from build123d import *

# Parameters (mm, degrees)
F0_W     = 170
F0_H     = 170
F0_R     = 1.98
F1_DEPTH = 1.57
F2_W     = 155
F2_H     = 27
F3_DEPTH = 39
F4_W     = 155
F4_H     = 30
F5_DEPTH = 38
F6_ANGLE = -90


with BuildPart() as f1:
    # F0 (on Front) → F1 (new body)
    with BuildSketch(Plane.XZ):
        with Locations((85, 85)):
            Rectangle(F0_W, F0_H)
        with Locations((6.35, 4.88)):
            Circle(F0_R, mode=Mode.SUBTRACT)
        with Locations((163.93, 4.88)):
            Circle(F0_R, mode=Mode.SUBTRACT)
        with Locations((6.35, 159.84)):
            Circle(F0_R, mode=Mode.SUBTRACT)
        with Locations((163.93, 147.14)):
            Circle(F0_R, mode=Mode.SUBTRACT)
    extrude(amount=F1_DEPTH)

    # F2 (on face) → F3 (join)
    with BuildSketch(Plane.XZ.offset(1.57)):
        with Locations((92.5, 156.5)):
            Rectangle(F2_W, F2_H)
    extrude(amount=F3_DEPTH)

    # F4 (on face) → F5 (join)
    with BuildSketch(Plane.XZ.offset(1.57)):
        with Locations((92.5, 15)):
            Rectangle(F4_W, F4_H)
    extrude(amount=F5_DEPTH)


with BuildPart() as f1_1:
    # F6: moved
    add(f1.part.rotate(Axis((0, -0.785, 0), (0, 1, 0)), F6_ANGLE))


with BuildPart() as f1_2:
    # F7: moved
    add(f1_1.part.moved(Location((170, 0, 0))))


solid = f1_2.part
Check sheet for the modelled part. Datum: model origin and axes. Units: mm. A direction names the side the tool comes from. Give positions to 0.01 mm unless a question says otherwise; leave off trailing zeros. Write each loop counter-clockwise with the first axis right and the second up, starting at its lowest first coordinate (ties: lowest second). Pieces come first, ordered by that corner, then holes. Notation, with made-up numbers: (19.25, 76) -> (45.25, 76) arc R11 ccw to (45.25, 89) -> close; hole circle Ø1 at (-4.75, 50). An arc over 180 degrees is marked (long way). One line per item, written item: value. Start each with the question number.
Item 1: Section check B-B on y = -17.5. Record the cut outline in (x, z).
Item 2: Draft check along Z on faces 4 (the flat face through (92, -1, 170)), 5 (the flat face through (84, -1.57, 84)), 6 (the cylindrical face through (163.157, -0.774, 6.092)), 7 (the flat face through (155, -20, 15)). Enter one of: +Z half, -Z half, draft (parallel to the pull), parting line (faces both ways), or undercut.
Item 3: Section check C-C on z = 6.35. Record the cut outline in (x, y).
Item 4: Section check A-A on x = 165.12. Record the cut outline in (y, z), then the cut area to 3 significant figures.
Item 5: Material ranges on probe 1 along X at (y, z) = (-0.65, 163.93); probe 2 along Z at (x, y) = (165.12, -0.35); probe 3 along X at (y, z) = (-0.75, 6.35), recorded low to high. Write a range as from..to.
Item 6: Gauge pin test, flat ends, axial feed: pin 1 (8 mm diameter, centred on x = 85.5, y = -5, fed in from -Z); pin 2 (2 mm diameter, centred on x = 165, z = 163, fed in from +Y); pin 3 (6 mm diameter, centred on x = 68.5, z = 41, fed in from -Y); pin 4 (13.5 mm diameter, centred on x = 9, y = -17, fed in from -Z). Record the tip position at first contact, or that the pin passes through.
Item 7: Section check D-D on x = 22.86. Record the cut outline in (y, z), then the cut area to 3 significant figures.
Item 8: Tool access check on faces 1 (the flat face through (23, -1.57, 164)), 2 (the flat face through (140, -20, 91)), 3 (the flat face through (155, -39.57, 91)). Record the directions out of +Z, -Z, +X, -X, +Y, -Y that give a thin tool (end or side, any length) a straight path to the whole face; none if there is none.
Results list:
1. outline: (0, 15) -> (27, 15) -> (27, 170) -> (0, 170) -> close; (140, 15) -> (170, 15) -> (170, 170) -> (140, 170) -> close
2. face 4: +Z half
2. face 5: draft
2. face 6: undercut
2. face 7: -Z half
3. outline: (0, -1.57) -> (8.18, -1.57) -> (8.18, 0) -> (0, 0) -> close; (12.14, -1.57) -> (163.14, -1.57) -> (163.14, 0) -> (12.14, 0) -> close; (167.1, -1.57) -> (170, -1.57) -> (170, 0) -> (167.1, 0) -> close
4. outline: (-39.57, 15) -> (-1.57, 15) -> (-1.57, 8.33) -> (0, 8.33) -> (0, 161.95) -> (-1.57, 161.95) -> (-1.57, 165.91) -> (0, 165.91) -> (0, 170) -> (-39.57, 170) -> close; (-1.57, 0) -> (0, 0) -> (0, 4.37) -> (-1.57, 4.37) -> close
4. area: 6,140 mm²
5. probe 1: 0..20.88, 24.84..163.14, 167.1..170
5. probe 2: 0..4.37, 8.33..161.95, 165.91..170
5. probe 3: 0..8.18, 12.14..163.14, 167.1..170
6. pin 1: z = 0
6. pin 2: y = -1.57
6. pin 3: y = -1.57
6. pin 4: z = 15
7. outline: (-40.57, 15) -> (-1.57, 15) -> (-1.57, 0) -> (0, 0) -> (0, 161.95) -> (-1.57, 161.95) -> (-1.57, 165.91) -> (0, 165.91) -> (0, 170) -> (-40.57, 170) -> close
7. area: 6,310 mm²
8. face 1: +Y
8. face 2: +Z, -Z, -Y
8. face 3: +Z, -Z, +X, -Y
